from build123d import *

# Parameters (mm, degrees)
EXTRUDE_1_DEPTH     = 236
CUT_EXTRUDE_1_DEPTH = 241.199916736


with BuildPart() as part:
    # Эскиз1 → Бобышка-Вытянуть1 (new body)
    with BuildSketch(Plane.XY):
        with BuildLine():
            Line((-18, 20), (18, 20))
            ThreePointArc((18, 20), (19.414213562, 19.414213562), (20, 18))
            Line((20, 18), (20, -18))
            ThreePointArc((20, -18), (19.414213562, -19.414213562), (18, -20))
            Line((18, -20), (-18, -20))
            ThreePointArc((-18, -20), (-19.414213562, -19.414213562), (-20, -18))
            Line((-20, -18), (-20, 18))
            ThreePointArc((-20, 18), (-19.414213562, 19.414213562), (-18, 20))
        make_face()
        with BuildLine():
            Line((-16, 18), (16, 18))
            ThreePointArc((16, 18), (17.414213562, 17.414213562), (18, 16))
            Line((18, 16), (18, -16))
            ThreePointArc((18, -16), (17.414213562, -17.414213562), (16, -18))
            Line((16, -18), (-16, -18))
            ThreePointArc((-16, -18), (-17.414213562, -17.414213562), (-18, -16))
            Line((-18, -16), (-18, 16))
            ThreePointArc((-18, 16), (-17.414213562, 17.414213562), (-16, 18))
        make_face(mode=Mode.SUBTRACT)
    extrude(amount=EXTRUDE_1_DEPTH)

    # Эскиз2 → Вырез-Вытянуть1 (cut, through all)
    with BuildSketch(Plane(origin=(0, 20, 0), x_dir=(1, 0, 0), z_dir=(0, 1, 0))):
        Polygon((20, -6), (-20, 0), (20, 0), align=None)
    extrude(amount=-CUT_EXTRUDE_1_DEPTH, mode=Mode.SUBTRACT)


solid = part.part
The model under review builds one solid part; all positions refer to its coordinate system, in mm. A direction names the side the tool comes from. Round coordinates to 2 decimals unless told otherwise and drop trailing zeros. Loops run counter-clockwise (first coordinate to the right, second up) from the corner with the lowest first, then second, coordinate; pieces in that order, holes last. Notation, with made-up numbers: (75.5, -30.75) -> (85.5, -30.75) arc R36 ccw to (85.5, 3.25) -> close; hole circle Ø1 at (35, 83.5). An arc over 180 degrees is marked (long way). Write item = value, one per line. Start each with the question number.
Item 1: Mouldability with a two-part tool opening along X and no side actions: class faces 3 (the flat face through (20, 0, 119)), 4 (the flat face through (-18, 0, 117)), 5 (the flat face through (0, 20, 117)) as released by +X, released by -X, zero draft, split by the parting line, or undercut.
Item 2: For faces 1 (the flat face through (0, 18, 117)), 2 (the flat face through (0, -20, 117)), list the 3-axis set-ups (+Z, -Z, +X, -X, +Y, -Y) from which the entire face can be reached by the end or side of a thin tool; tool diameter is ignored.
Item 3: Take a section at B-B on y = -3.5. Give the boundary of the cut face in (x, z), plus the area to 3 significant figures.
Item 4: To check wall thickness, follow L1, parallel to X at y = 3, z = 61.5; L2, parallel to Y at x = -16.5, z = 142. State the ranges of each line that lie inside material, in increasing order.
Item 5: Take a section at A-A on x = -5. Give the boundary of the cut face in (y, z), plus the area to 3 significant figures.
Item 6: Take a section at C-C on z = 139. Give the boundary of the cut face in (x, y).
Item 7: Insertion check: pin 1 (10 mm diameter, centred on x = -5, y = 13.5, fed in from -Z); pin 2 (10 mm diameter, centred on x = 6.5, y = 15.5, fed in from +Z); pin 3 (8 mm diameter, centred on x = 7, y = -11, fed in from -Z). Each pin has a flat end and moves straight along its axis. Give the tip position at first contact, or say it passes through.
Result:
q1.face_3 = released by +X
q1.face_4 = undercut
q1.face_5 = zero draft
q2.face_1 = +Z, -Z
q2.face_2 = +Z, -Z, +X, -X, -Y
q3.outline = (-20, 0) -> (-18, 0.3) -> (-18, 236) -> (-20, 236) -> close; (18, 5.7) -> (20, 6) -> (20, 236) -> (18, 236) -> close
q3.area = 932 mm²
q4.L1 = -20 to -18, 18 to 20
q4.L2 = -20 to -17.94, 17.94 to 20
q5.outline = (-20, 2.25) -> (-18, 2.25) -> (-18, 236) -> (-20, 236) -> close; (18, 2.25) -> (20, 2.25) -> (20, 236) -> (18, 236) -> close
q5.area = 935 mm²
q6.outline = (-20, -18) arc R2 ccw to (-18, -20) -> (18, -20) arc R2 ccw to (20, -18) -> (20, 18) arc R2 ccw to (18, 20) -> (-18, 20) arc R2 ccw to (-20, 18) -> close; hole (-18, -16) arc R2 ccw to (-16, -18) -> (16, -18) arc R2 ccw to (18, -16) -> (18, 16) arc R2 ccw to (16, 18) -> (-16, 18) arc R2 ccw to (-18, 16) -> close
q7.pin_1 = 1.92
q7.pin_2 = 236
q7.pin_3 = through
